Build history of the part. All positions in model axes, mm. Face numbers are marked on the shaded views. Give positions to 0.01 mm unless a question says otherwise; leave off trailing zeros. Order: outer loops, then holes, each group sorted by start corner. A loop starts at its lowest first (then second) coordinate and runs counter-clockwise, first axis right, second up. Notation, with made-up numbers: (-15.5, -27.5) - (-5.5, -27.5) arc R32 ccw to (-5.5, 4.5) - close; hole circle Ø3 at (30, 53). An arc over 180 degrees is marked (long way). Use a Markdown table: item, result.
from build123d import *

# Parameters (mm, degrees)
SKETCH1_W               = 140.97
SKETCH1_H               = 144.78
BOSS_EXTRUDE1_DEPTH     = 5.08
SKETCH2_W               = 140.97
SKETCH2_H               = 144.78
SKETCH2_W_2             = 115.57
SKETCH2_H_2             = 12.7
SKETCH2_W_3             = 130.81
SKETCH2_H_3             = 120.65
BOSS_EXTRUDE2_DEPTH     = 5.55625
SKETCH3_W               = 115.57
SKETCH3_H               = 19.05
CUT_EXTRUDE1_DEPTH      = 3.175
SKETCH4_R               = 2.2
BOSS_EXTRUDE3_DEPTH     = 3
MIRROR2_COPY_1_SKETCH_R = 2.2
MIRROR2_COPY_1_DEPTH    = 3
SKETCH5_R               = 2.2
CUT_EXTRUDE2_DEPTH      = 109.755169743
SKETCH6_R               = 4.572
CUT_EXTRUDE3_DEPTH      = 2.54
FILLET1_R               = 3.81


with BuildPart() as part:
    # Sketch1 → Boss-Extrude1 (new body)
    with BuildSketch(Plane(origin=(0, 0, 0), x_dir=(1, 0, 0), z_dir=(0, 1, 0))):
        Rectangle(SKETCH1_W, SKETCH1_H)
    extrude(amount=BOSS_EXTRUDE1_DEPTH)

    # Sketch2 → Boss-Extrude2 (add)
    with BuildSketch(Plane.XZ):
        Rectangle(SKETCH2_W, SKETCH2_H)
        with Locations((0, 62.865)):
            Rectangle(SKETCH2_W_2, SKETCH2_H_2, mode=Mode.SUBTRACT)
        with Locations((0, -6.985)):
            Rectangle(SKETCH2_W_3, SKETCH2_H_3, mode=Mode.SUBTRACT)
    extrude(amount=BOSS_EXTRUDE2_DEPTH)

    # Sketch3 → Cut-Extrude1 (cut)
    with BuildSketch(Plane.XZ.offset(5.55625)):
        with Locations((0, 62.865)):
            Rectangle(SKETCH3_W, SKETCH3_H)
    extrude(amount=-CUT_EXTRUDE1_DEPTH, mode=Mode.SUBTRACT)

    # Sketch4 → Boss-Extrude3 (add)
    with BuildSketch(Plane(origin=(57.785, 0, 0), x_dir=(0, 0, -1), z_dir=(1, 0, 0))):
        with BuildLine():
            Line((72.39, 5.08), (80.298586194, -2.669654518))
            ThreePointArc((80.298586194, -2.669654518), (80.144596616, -8.586079413), (74.254776903, -8.004856495))
            Line((74.254776903, -8.004856495), (72.39, -5.55625))
            Line((72.39, -5.55625), (72.39, 5.08))
        make_face()
        with Locations((77.47, -5.55625)):
            Circle(SKETCH4_R, mode=Mode.SUBTRACT)
    boss_extrude3 = extrude(amount=-BOSS_EXTRUDE3_DEPTH)

    # Mirror1: Boss-Extrude3 across plane
    add(boss_extrude3.mirror(Plane.ZY.offset(-51.784999904)))

    # Mirror2: Boss-Extrude3 across plane
    add(boss_extrude3.mirror(Plane(origin=(0, 0, 0), x_dir=(0, 0, 1), z_dir=(1, 0, 0))))

    # Mirror2 copy 1 sketch → Mirror2 copy 1 (add)
    with BuildSketch(Plane(origin=(-45.784999808, 0, 0), x_dir=(0, 0, -1), z_dir=(1, 0, 0))):
        with BuildLine():
            Line((72.39, 5.08), (80.298586194, -2.669654518))
            ThreePointArc((80.298586194, -2.669654518), (80.144596616, -8.586079413), (74.254776903, -8.004856495))
            Line((74.254776903, -8.004856495), (72.39, -5.55625))
            Line((72.39, -5.55625), (72.39, 5.08))
        make_face()
        with Locations((77.47, -5.55625)):
            Circle(MIRROR2_COPY_1_SKETCH_R, mode=Mode.SUBTRACT)
    extrude(amount=-MIRROR2_COPY_1_DEPTH)

    # Sketch5 → Cut-Extrude2 (cut, through all)
    with BuildSketch(Plane(origin=(0, 5.08, 0), x_dir=(1, 0, 0), z_dir=(0, 1, 0))):
        with Locations(Location((64.008, -62.865, 0), (0, 0, 270))):
            Circle(SKETCH5_R)
        with Locations(Location((-64.008, -62.865, 0), (0, 0, 270))):
            Circle(SKETCH5_R)
    extrude(amount=-CUT_EXTRUDE2_DEPTH, mode=Mode.SUBTRACT)

    # Sketch6 → Cut-Extrude3 (cut)
    with BuildSketch(Plane.XZ.offset(5.55625)):
        with Locations(Location((-64.008, 62.865, 0), (0, 0, 270))):
            Circle(SKETCH6_R)
        with Locations(Location((64.008, 62.865, 0), (0, 0, 270))):
            Circle(SKETCH6_R)
    extrude(amount=-CUT_EXTRUDE3_DEPTH, mode=Mode.SUBTRACT)

    # Fillet1
    fillet1_edges = [part.edges().sort_by_distance(p)[0] for p in [
        (-70.485, 5.08, 0),
        (0, 5.08, 72.39),
        (70.485, 5.08, 0),
        (70.485, -0.238125, 72.39),
        (-70.485, -0.238125, 72.39),
        (-70.485, -0.238125, -72.39),
        (70.485, -0.238125, -72.39),
    ]]
    fillet(fillet1_edges, radius=FILLET1_R)


solid = part.part
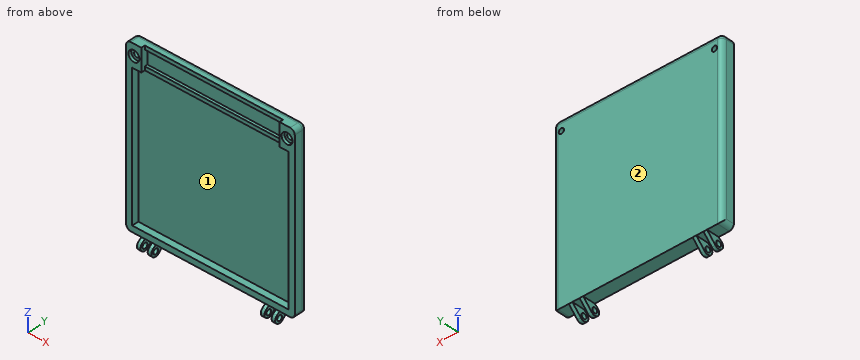
1) Wall check: line 1 (Z direction, x = 39, y = -1.25) (3 decimals); line 2 (X direction, y = -0.75, z = -58.5) (3 decimals); line 3 (Z direction, x = 2.5, y = -5.5). Give the ranges that are in metal, low to high. Write a range as from..to.
Computed:
| item | result |
|---|---|
| line 1 | z = -72.39..-67.31, 53.34..56.515, 69.215..72.39 |
| line 2 | x = -70.485..-65.405, 65.405..70.485 |
| line 3 | z = -72.39..-67.31 |
2) Pin check, flat tips, straight feed: P1, Ø14, axis at x = -20.5, z = 61, coming from the -Y side; P2, Ø1.2, axis at x = -2.5, y = -1.5, coming from the -Z side; P3, Ø10, axis at x = -64, z = 63, coming from the -Y side; P4, Ø14.5, axis at x = 64.008, z = 62.865, coming from the +Y side. Stop position of each tip, or through.
Computed:
| item | result |
|---|---|
| P1 | stops at y = -2.38 |
| P2 | stops at z = -72.39 |
| P3 | stops at y = -5.56 |
| P4 | stops at y = 5.08 |
3) Slice it at C-C (z = 24). Write the cut outline in (x, y) (3 decimals).
Computed:
| item | result |
|---|---|
| outline | (-70.485, -5.556) - (-65.405, -5.556) - (-65.405, 0) - (65.405, 0) - (65.405, -5.556) - (70.485, -5.556) - (70.485, 1.27) arc R3.81 ccw to (66.675, 5.08) - (-66.675, 5.08) arc R3.81 ccw to (-70.485, 1.27) - close |
4) Two-plate mould, pull along Z, no slides. Class the marked faces 1 and 2: +Z half, -Z half, draft (parallel to the pull), parting line (faces both ways), or undercut.
Computed:
| item | result |
|---|---|
| face 1 | undercut |
| face 2 | draft |
5) Slice it at B-B (x = -34). Write the cut outline in (y, z) (3 decimals), and give its area (3 significant figures).
Computed:
| item | result |
|---|---|
| outline | (-5.556, -72.39) - (5.08, -72.39) - (5.08, 68.58) arc R3.81 ccw to (1.27, 72.39) - (-2.381, 72.39) - (-2.381, 69.215) - (0, 69.215) - (0, 56.515) - (-2.381, 56.515) - (-2.381, 53.34) - (0, 53.34) - (0, -67.31) - (-5.556, -67.31) - close |
| area | 776 mm² |
6) Slice it at A-A (z = -77.47). State how many separate pieces and enclosed holes the cut face has, and give its area (3 significant figures).
Computed:
| item | result |
|---|---|
| separate pieces | 8 |
| enclosed holes | 0 |
| area | 63.6 mm² |
